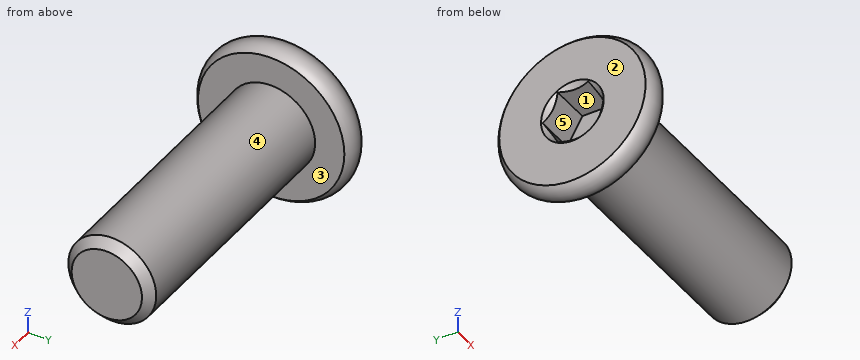
from build123d import *

# Parameters (mm, degrees)
SKETCH2_R           = 2.5
BOSS_EXTRUDE1_DEPTH = 15
CHAMFER1_SIZE       = 0.5
CUT_EXTRUDE1_DEPTH  = 2.3
SKETCH8_R           = 1.782050808
CUT_EXTRUDE2_DEPTH  = 1
CUT_EXTRUDE2_TAPER  = 45


with BuildPart() as part:
    # Sketch2 → Boss-Extrude1 (new body)
    with BuildSketch(Plane(origin=(0, 0, 0), x_dir=(0, 0, -1), z_dir=(1, 0, 0))):
        Circle(SKETCH2_R)
    extrude(amount=-BOSS_EXTRUDE1_DEPTH)

    # Chamfer1
    chamfer1_edges = [part.edges().sort_by_distance(p)[0] for p in [
        (0, 0, 2.5),
    ]]
    chamfer(chamfer1_edges, length=CHAMFER1_SIZE)

    # Sketch6 → Revolve1 (revolve)
    with BuildSketch(Plane.XY):
        with BuildLine():
            Line((-16.5, 0), (-16.5, 4.161437828))
            ThreePointArc((-16.5, 4.161437828), (-15.75, 4.5), (-15, 4.161437828))
            Line((-15, 4.161437828), (-15, 0))
            Line((-15, 0), (-16.5, 0))
        make_face()
    revolve(axis=Axis((-15, 0, 0), (1, 0, 0)))

    # Sketch7 → Cut-Extrude1 (cut)
    with BuildSketch(Plane.ZY.offset(16.5)):
        Polygon((0, 1.732050808), (-1.5, 0.866025404), (-1.5, -0.866025404), (0, -1.732050808), (1.5, -0.866025404), (1.5, 0.866025404), align=None)
    extrude(amount=-CUT_EXTRUDE1_DEPTH, mode=Mode.SUBTRACT)

    # Sketch8 → Cut-Extrude2 (cut)
    with BuildSketch(Plane.ZY.offset(16.5)):
        Circle(SKETCH8_R)
    extrude(amount=-CUT_EXTRUDE2_DEPTH, taper=CUT_EXTRUDE2_TAPER, mode=Mode.SUBTRACT)


solid = part.part
The listing builds one solid part. Answer for the finished solid, in the listing's coordinates (mm). Face numbers are marked on the shaded views. A direction names the side the tool comes from. Coordinates: 2 decimals unless noted, no trailing zeros. Order: outer loops, then holes, each group sorted by start corner. A loop starts at its lowest first (then second) coordinate and runs counter-clockwise, first axis right, second up. Notation, with made-up numbers: (-18.75, -20.5) -> (38.25, -20.5) arc R26 ccw to (38.25, 0.5) -> close; hole circle Ø9 at (-36, 78.5). An arc over 180 degrees is marked (long way). Answer in a Markdown table with one row per item. Add a question column.
Item 1: Find the intervals of material crossed by L1, parallel to Z at x = -3, y = 2; L2, parallel to Y at x = -7, z = -1.75; L3, parallel to X at y = 1, z = 4, in increasing order. Write a range as from..to.
Item 2: Each of these flat-tipped pins is pushed along its axis until it touches: P1, Ø1.5, axis at y = -0.5, z = 0.5, coming from the -X side; P2, Ø4, axis at x = -14, y = 3.5, coming from the +Z side; P3, Ø1.5, axis at x = -8, z = -3.5, coming from the -Y side; P4, Ø1.5, axis at x = -10, z = 0.5, coming from the -Y side. Where does it stop, or does it pass through?
Item 3: Find section A-A (x = -9.5). Write down the section's boundary in (y, z), then the cut area to 3 significant figures.
Item 4: Determine the mould class of the marked faces 3, 4 and 5 for opening direction Z: +Z half, -Z half, draft (parallel to the pull), parting line (faces both ways), or undercut.
Item 5: Which of the six approach directions +Z, -Z, +X, -X, +Y, -Y give full straight-line access (tool end or side, diameter ignored) to the marked faces 1 and 2?
Result set:
| question | item | result |
|---|---|---|
| 1 | L1 | z = -1.5..1.5 |
| 1 | L2 | y = -1.79..1.79 |
| 1 | L3 | x = -16.5..-15 |
| 2 | P1 | stops at x = -14.2 |
| 2 | P2 | stops at z = 3.93 |
| 2 | P3 | passes through |
| 2 | P4 | stops at y = -2.5 |
| 3 | outline | circle Ø5 at (0, 0) |
| 3 | area | 19.6 mm² |
| 4 | face 3 | draft |
| 4 | face 4 | parting line |
| 4 | face 5 | undercut |
| 5 | face 1 | -X |
| 5 | face 2 | +Z, -Z, -X, +Y, -Y |
